Study the drawing (mm; zero at the part's minimum x, y, z) and answer. A direction names the side the tool comes from. Coordinates: 2 decimals unless noted, no trailing zeros. Order: outer loops, then holes, each group sorted by start corner. A loop starts at its lowest first (then second) coordinate and runs counter-clockwise, first axis right, second up.
1. Flat-ended cylindrical pins translate along their axes: pin 1 Ø1 at (x, z) = (13, 40.5) entering from +Y; pin 2 Ø4 at (x, z) = (68.5, 30) entering from +Y; pin 3 Ø5 at (x, z) = (37.5, 24.5) entering from +Y (1 decimal). Find the tip coordinate at first contact, or state that the pin passes through.
2. Determine the mould class of the marked faces 3, 4 and 5 for opening direction Z: +Z half, -Z half, draft (parallel to the pull), parting line (faces both ways), or undercut.
3. A tool of negligible diameter and unlimited length cuts with its end or side. For the marked faces 1 and 2, from which of +Z, -Z, +X, -X, +Y, -Y can it reach the whole face along a straight path? Write none if from no direction.
4. The part is cut by section D-D, the plane x = 20. Give the vertices of the cut face in (y, z), then the cut area to 3 significant figures.
5. Find the intervals of material crossed by probe 1 along Z at (x, y) = (68.5, 30); probe 2 along Z at (x, y) = (7.75, 30), in increasing order.
6. The part is cut by section A-A, the plane y = 30. Give the vertices of the cut face in (x, z), then the cut area to 3 significant figures.
7. The part is cut by section C-C, the plane x = 57. Give the vertices of the cut face in (y, z).
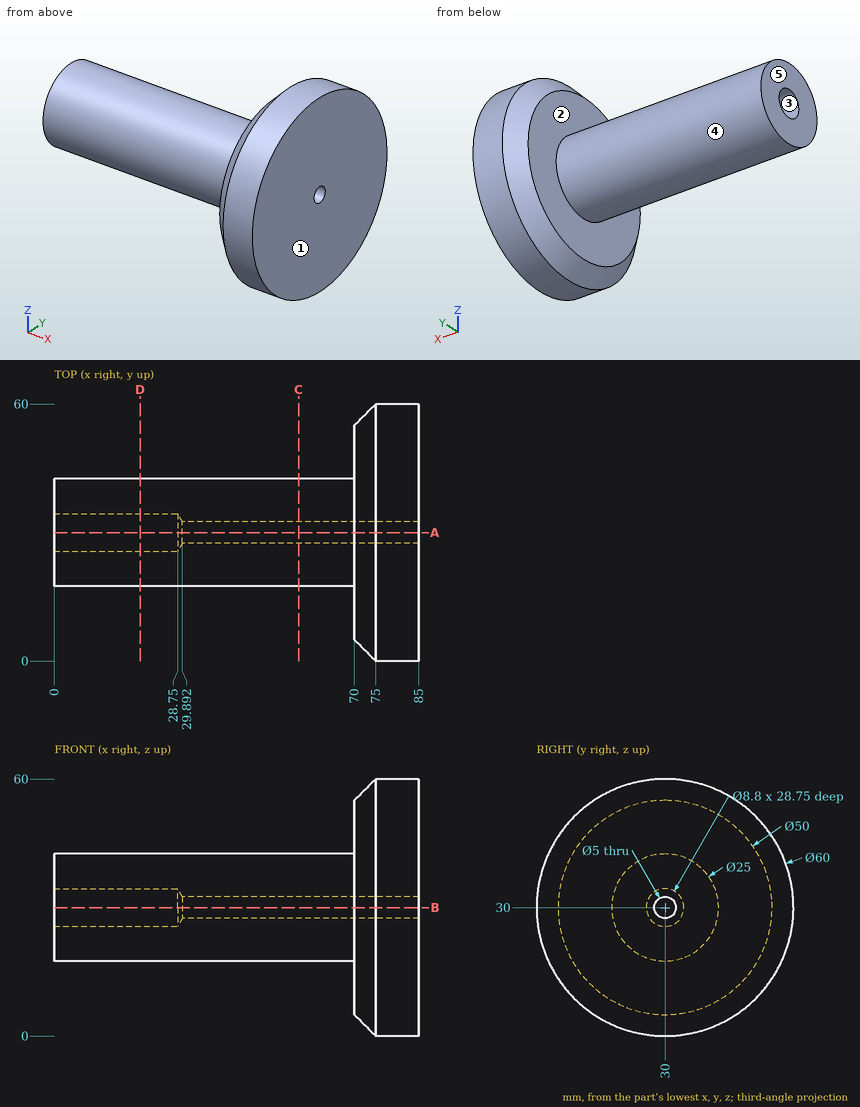
Geometry says:
1. pin 1: stops at y = 37.5
1. pin 2: stops at y = 55.5
1. pin 3: stops at y = 42.1
2. face 3: undercut
2. face 4: parting line
2. face 5: draft
3. face 1: +Z, -Z, +X, +Y, -Y
3. face 2: -X
4. outline: circle Ø25 at (30, 30); hole circle Ø8.8 at (30, 30)
4. area: 430 mm2
5. probe 1: z = 17.5 to 27.5, 32.5 to 42.5
5. probe 2: z = 17.5 to 25.6, 34.4 to 42.5
6. outline: (0, 17.5) - (70, 17.5) - (70, 5) - (75, 0) - (85, 0) - (85, 27.5) - (29.89, 27.5) - (28.75, 25.6) - (0, 25.6) - close; (0, 34.4) - (28.75, 34.4) - (29.89, 32.5) - (85, 32.5) - (85, 60) - (75, 60) - (70, 55) - (70, 42.5) - (0, 42.5) - close
6. area: 2,090 mm2
7. outline: circle Ø25 at (30, 30); hole circle Ø5 at (30, 30)
